Answer from the drawing. Dimensions are ordinates in mm from the lowest x, y and z of the part. A direction names the side the tool comes from. Round coordinates to 2 decimals unless told otherwise and drop trailing zeros. Write each loop counter-clockwise with the first axis right and the second up, starting at its lowest first coordinate (ties: lowest second). Pieces come first, ordered by that corner, then holes. Notation, with made-up numbers: (70.5, -10.75) -> (111.5, -10.75) arc R18 cw to (111.5, 23.25) -> close; hole circle Ø9 at (4, 56). An arc over 180 degrees is marked (long way). Return JSON: item names as keys, results as strings. Group by question number.
(1) Straight lines are drawn through the part: line 1 (X direction, y = 36, z = 32); line 2 (Z direction, x = 206, y = 137.5); line 3 (X direction, y = 83, z = 29). For each, find the intervals that lie inside material, in ascending order.
(2) For the marked faces 1, 2, 3 and 4, determine the directions among +Z, -Z, +X, -X, +Y, -Y from which every point of the face is accessible in a straight line to the end or side of a thin tool.
(3) Given pin 1 (7.5 mm diameter, centred on y = 64, z = 18, fed in from +X); pin 2 (1 mm diameter, centred on x = 209.5, y = 129.5, fed in from +Z); pin 3 (8 mm diameter, centred on x = 140.5, y = 110, fed in from +Z), each flat-ended and moving along its own axis, determine where each tip first touches the part or whether it passes through.
(4) A cutting plane is placed at B-B on z = 76.2. Give the vertices of the cut face in (x, y), then the cut area to 3 significant figures.
(5) A cutting plane is placed at D-D on z = 43.5. Give the vertices of the cut face in (x, y), then the cut area to 3 significant figures.
(6) A cutting plane is placed at A-A on y = 101.6. Give the vertices of the cut face in (x, z), then the cut area to 3 significant figures.
(7) A cutting plane is placed at C-C on y = 183.5. Give the vertices of the cut face in (x, z).
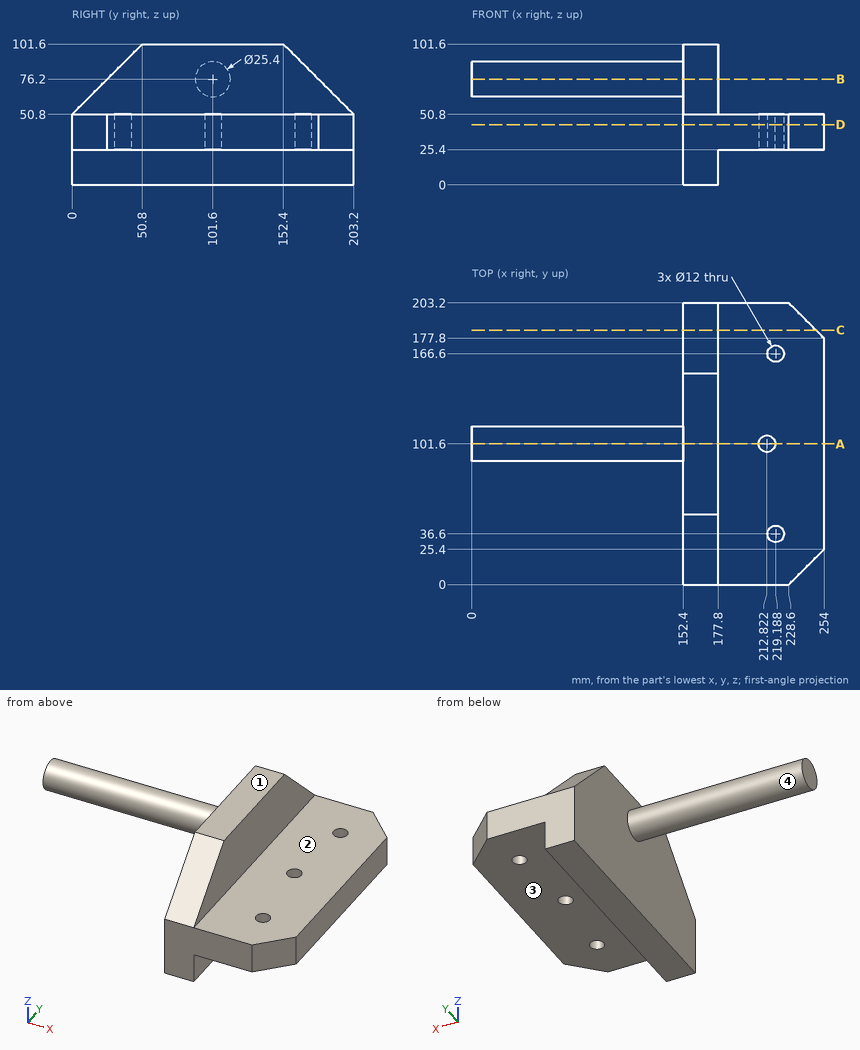
Checks:
{
 "1": {"line 1": "x = 152.4 to 213.22, 225.16 to 254", "line 2": "z = 25.4 to 50.8", "line 3": "x = 152.4 to 254"},
 "2": {"face 1": "+Z, +X, -X, +Y, -Y", "face 2": "+Z, +X, +Y, -Y", "face 3": "-Z, +X, +Y, -Y", "face 4": "-X"},
 "3": {"pin 1": "stops at x = 177.8", "pin 2": "stops at z = 50.8", "pin 3": "stops at z = 88.11"},
 "4": {"outline": "(0, 88.9) -> (152.4, 88.9) -> (152.4, 25.4) -> (177.8, 25.4) -> (177.8, 177.8) -> (152.4, 177.8) -> (152.4, 114.3) -> (0, 114.3) -> close", "area": "7,740 mm^2"},
 "5": {"outline": "(152.4, 0) -> (228.6, 0) -> (254, 25.4) -> (254, 177.8) -> (228.6, 203.2) -> (152.4, 203.2) -> close; hole circle Ø12 at (212.82, 101.6); hole circle Ø12 at (219.19, 36.6); hole circle Ø12 at (219.19, 166.6)", "area": "19,700 mm^2"},
 "6": {"outline": "(0, 63.5) -> (152.4, 63.5) -> (152.4, 0) -> (177.8, 0) -> (177.8, 25.4) -> (206.82, 25.4) -> (206.82, 50.8) -> (177.8, 50.8) -> (177.8, 101.6) -> (152.4, 101.6) -> (152.4, 88.9) -> (0, 88.9) -> close; (218.82, 25.4) -> (254, 25.4) -> (254, 50.8) -> (218.82, 50.8) -> close", "area": "8,080 mm^2"},
 "7": {"outline": "(152.4, 0) -> (177.8, 0) -> (177.8, 25.4) -> (248.3, 25.4) -> (248.3, 50.8) -> (177.8, 50.8) -> (177.8, 70.5) -> (152.4, 70.5) -> close"}
}
